Could you check a few things on this model? Use its own coordinates, in mm. A direction names the side the tool comes from. Give positions to 0.01 mm unless a question says otherwise; leave off trailing zeros. Order: outer loops, then holes, each group sorted by start corner. A loop starts at its lowest first (then second) coordinate and runs counter-clockwise, first axis right, second up. Notation, with made-up numbers: (36.5, 79.25) -> (46.5, 79.25) arc R30 cw to (46.5, 112.25) -> close; hole circle Ø1 at (-3.5, -33). An arc over 180 degrees is marked (long way). Use one line per item in the form item = value. Start each with the question number.
from build123d import *

# Parameters (mm, degrees)
F0_R     = 3
F0_R_2   = 1.8
F1_DEPTH = 6
F2_DEPTH = 15
F3_DEPTH = 3
F4_R     = 3.875
F5_DEPTH = 2


with BuildPart() as f1:
    # F0 (on Top) → F1 (new body)
    with BuildSketch(Plane.XY):
        with BuildLine():
            Line((10.6606484084, -5.5091356412), (22.5, -5.5091356412))
            Line((22.5, -5.5091356412), (22.5, 20.5))
            Line((22.5, 20.5), (-22.5, 20.5))
            Line((-22.5, 20.5), (-22.5, -1.5091356412))
            Line((-22.5, -1.5091356412), (-14, -1.5091356412))
            Line((-14, -1.5091356412), (-14, 4.4908643588))
            Line((-14, 4.4908643588), (-12, 4.4908643588))
            Line((-12, 4.4908643588), (-12, 0))
            ThreePointArc((-12, 0), (0, 12), (12, 0))
            ThreePointArc((12, 0), (11.6603555027, -2.8348032647), (10.6606484084, -5.5091356412))
        make_face()
        with Locations((-15.5, 15.5)):
            Circle(F0_R, mode=Mode.SUBTRACT)
        with Locations((15.5, 15.5)):
            Circle(F0_R, mode=Mode.SUBTRACT)
        Polygon((-14, -1.5091356412), (-22.5, -1.5091356412), (-22.5, -5.5091356412), (-12, -5.5091356412), (-12, 0), (-12, 4.4908643588), (-14, 4.4908643588), align=None)
        with Locations((15.5, 15.5)):
            Circle(F0_R)
        with Locations((15.5, 15.5)):
            Circle(F0_R_2, mode=Mode.SUBTRACT)
    extrude(amount=F1_DEPTH)

    # F0 (on Top) → F2 (join)
    with BuildSketch(Plane.XY):
        Polygon((-14, -1.5091356412), (-22.5, -1.5091356412), (-22.5, -5.5091356412), (-12, -5.5091356412), (-12, 0), (-12, 4.4908643588), (-14, 4.4908643588), align=None)
        with BuildLine():
            Line((-12, -5.5091356412), (-10.6606484084, -5.5091356412))
            ThreePointArc((-10.6606484084, -5.5091356412), (-11.6603555027, -2.8348032647), (-12, 0))
            Line((-12, 0), (-12, -5.5091356412))
        make_face()
    extrude(amount=F2_DEPTH)

    # F0 (on Top) → F3 (join)
    with BuildSketch(Plane.XY):
        with Locations((-15.5, 15.5)):
            Circle(F0_R)
        with Locations((-15.5, 15.5)):
            Circle(F0_R_2, mode=Mode.SUBTRACT)
    extrude(amount=F3_DEPTH)

    # F4 (on face) → F5 (cut)
    with BuildSketch(Plane(origin=(0, -1.5091356412, 0), x_dir=(-1, 0, 0), z_dir=(0, 1, 0))):
        with Locations((18.25, 10.5)):
            Circle(F4_R)
    extrude(amount=-F5_DEPTH, mode=Mode.SUBTRACT)


solid = f1.part
(1) Which directions (+Z, -Z, +X, -X, +Y, -Y) give clear straight access to the entire face, cutting with the end or side of a thin tool? Please do faces 4 (the flat face through (-15, -1.509, 13)), 5 (the flat face through (-13, 4.491, 10)), 6 (the flat face through (-18, -3.509, 11)), 7 (the cylindrical face through (-16.15, 12.57, 4.48)).
(2) Imagine slicing it at B-B (z = 3.5). Write out the boundary of the cut face in (x, y), plus the area to 3 significant figures.
(3) Imagine slicing it at C-C (y = 8.75). Write out the boundary of the cut face in (x, z), plus the area to 3 significant figures.
(4) We'd pull the mould along X, two halves only. Please class faces 1 (the flat face through (-17, -3, 15)), 2 (the flat face through (-12, 2, 10)), 3 (the flat face through (-14, 14, 3)): pulls with the +X half, pulls with the -X half, needs draft (parallel to the pull), parting line crosses it, or undercut.
(5) Please list where these lines run through material, in increasing order: probe 1 along Y at (x, z) = (-15.5, 1.8); probe 2 along Z at (x, y) = (-18.25, -2.75) (3 decimals); probe 3 along Y at (x, z) = (-15.5, 4.35).
(6) Imagine slicing it at A-A (x = 15.5). Write out the boundary of the cut face in (y, z), plus the area to 3 significant figures.
(7) I'm going to push flat-ended pins straight in: pin 1 Ø4 at (x, z) = (-16.5, 11) entering from +Y; pin 2 Ø3.5 at (y, z) = (1.5, 8.5) entering from +X; pin 3 Ø4.5 at (x, y) = (15.5, 15.5) entering from +Z. Where does each tip first touch, or does it pass through?
(8) Imagine slicing it at D-D (z = 10.5). Write out the boundary of the cut face in (x, y) (3 decimals), plus the area to 3 significant figures.
Calculated:
q1.face_4 = +Z, -X, +Y
q1.face_5 = +Z, +X, -X, +Y
q1.face_6 = +Y
q1.face_7 = +Z
q2.outline = (-22.5, -5.51) -> (-10.66, -5.51) arc R12 cw (long way) to (10.66, -5.51) -> (22.5, -5.51) -> (22.5, 20.5) -> (-22.5, 20.5) -> close; hole circle Ø6 at (-15.5, 15.5); hole circle Ø3.6 at (15.5, 15.5)
q2.area = 778 mm2
q3.outline = (-22.5, 0) -> (-8.21, 0) -> (-8.21, 6) -> (-22.5, 6) -> close; (8.21, 0) -> (22.5, 0) -> (22.5, 6) -> (8.21, 6) -> close
q3.area = 171 mm2
q4.face_1 = needs draft
q4.face_2 = pulls with the +X half
q4.face_3 = undercut
q5.probe_1 = -5.51 to 13.7, 17.3 to 20.5
q5.probe_2 = 0 to 6.625, 14.375 to 15
q5.probe_3 = -5.51 to 12.5, 18.5 to 20.5
q6.outline = (-5.51, 0) -> (13.7, 0) -> (13.7, 6) -> (-5.51, 6) -> close; (17.3, 0) -> (20.5, 0) -> (20.5, 6) -> (17.3, 6) -> close
q6.area = 134 mm2
q7.pin_1 = -3.51
q7.pin_2 = -12
q7.pin_3 = 6
q8.outline = (-22.5, -5.509) -> (-10.661, -5.509) arc R12 cw to (-12, 0) -> (-12, 4.491) -> (-14, 4.491) -> (-14, -1.509) -> (-14.375, -1.509) -> (-14.375, -3.509) -> (-22.125, -3.509) -> (-22.125, -1.509) -> (-22.5, -1.509) -> close
q8.area = 40.9 mm2
